Drawing for the job (mm, zero at the part's lowest x, y, z). A direction names the side the tool comes from. Round coordinates to 2 decimals unless told otherwise and drop trailing zeros. Loops run counter-clockwise (first coordinate to the right, second up) from the corner with the lowest first, then second, coordinate; pieces in that order, holes last. Notation, with made-up numbers: M 19,43.25 L 59,43.25 A14 ccw 59,64.25 Z; hole C -36.75,64.5 d5. An arc over 180 degrees is marked long. Answer in a Markdown table with one row per item.
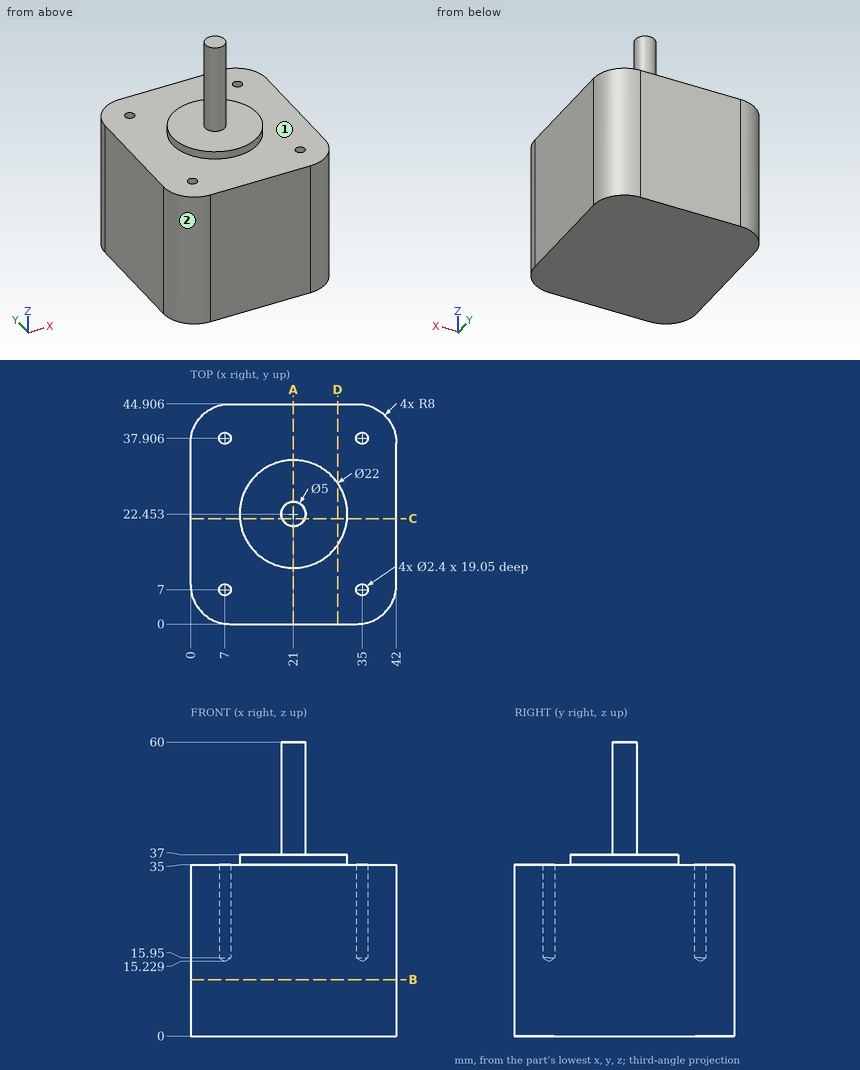
1. Saw through at C-C (y = 21.5). Write the cut outline in (x, z).
Verdict:
| item | result |
|---|---|
| outline | M 0,0 L 42,0 L 42,35 L 31.96,35 L 31.96,37 L 23.31,37 L 23.31,60 L 18.69,60 L 18.69,37 L 10.04,37 L 10.04,35 L 0,35 Z |
2. Pin check, flat tips, straight feed: pin 1 (1.5 mm diameter, centred on x = 17.5, y = 13.5, fed in from +Z); pin 2 (8 mm diameter, centred on y = 13, z = 47.5, fed in from -X); pin 3 (3 mm diameter, centred on x = 16, y = 36, fed in from +Z); pin 4 (1 mm diameter, centred on y = 22, z = 41, fed in from +X). Stop position of each tip, or through.
Verdict:
| item | result |
|---|---|
| pin 1 | stops at z = 37 |
| pin 2 | passes through |
| pin 3 | stops at z = 35 |
| pin 4 | stops at x = 23.5 |
3. Saw through at D-D (x = 30). Write the cut outline in (y, z) (1 decimal), and give its area (3 significant figures).
Verdict:
| item | result |
|---|---|
| outline | M 0,0 L 44.9,0 L 44.9,35 L 28.8,35 L 28.8,37 L 16.1,37 L 16.1,35 L 0,35 Z |
| area | 1,600 mm² |
4. Wall check: probe 1 along X at (y, z) = (7, 25.25); probe 2 along Y at (x, z) = (7, 24) (1 decimal); probe 3 along Z at (x, y) = (26, 35.5). Give the ranges that are in metal, low to high.
Verdict:
| item | result |
|---|---|
| probe 1 | x = 0.06 to 5.8, 8.2 to 33.8, 36.2 to 41.94 |
| probe 2 | y = 0.1 to 5.8, 8.2 to 36.7, 39.1 to 44.8 |
| probe 3 | z = 0 to 35 |
5. Saw through at B-B (z = 11.5). Write the cut outline in (x, y) (1 decimal), and give its area (3 significant figures).
Verdict:
| item | result |
|---|---|
| outline | M 0,8 A8 ccw 8,0 L 34,0 A8 ccw 42,8 L 42,36.9 A8 ccw 34,44.9 L 8,44.9 A8 ccw 0,36.9 Z |
| area | 1,830 mm² |
6. Saw through at A-A (x = 21). Write the cut outline in (y, z) (1 decimal).
Verdict:
| item | result |
|---|---|
| outline | M 0,0 L 44.9,0 L 44.9,35 L 33.5,35 L 33.5,37 L 25,37 L 25,60 L 20,60 L 20,37 L 11.5,37 L 11.5,35 L 0,35 Z |
7. Tool access for the marked faces 1 and 2: list every direction of +Z, -Z, +X, -X, +Y, -Y with a clear straight run to the whole face (end or side of a thin tool).
Verdict:
| item | result |
|---|---|
| face 1 | +Z |
| face 2 | +Z, -Z, -X, -Y |
